```python
from build123d import *

# Parameters (mm, degrees)
F1_DEPTH      = 203.2
F1_DEPTH_BACK = 203.2
F0_W          = 63.5
F0_H          = 101.6
F0_R          = 54
F2_DEPTH      = 127
F2_DEPTH_BACK = 127
F3_DEPTH      = 101.6
F3_DEPTH_BACK = 101.6
F4_DEPTH      = 152.4
F4_DEPTH_BACK = 114.3
F5_T1_DEPTH   = 825.5
F5_T6_DEPTH   = 825.5
F5_T11_DEPTH  = 444.5
F5_T16_DEPTH  = 825.5
F5_T21_DEPTH  = 825.5
F6_DEPTH      = 152.4
F6_DEPTH_BACK = 152.4
F7_R          = 165.1
F8_DEPTH      = 50.8


# Not quite as in the source:
# - a fillet or chamfer that OpenCascade refuses, or shapes differently, is made with other operations: its cross-section is extruded or revolved along the edge and cut away or added


with BuildPart() as f1:
    # F0 (on Right) → F1 (new body, two sides)
    with BuildSketch(Plane.YZ) as f1_sk:
        Polygon((-177.8, -50.8), (-114.3, -50.8), (-114.3, 292.1), (-114.3, 330.2), (-177.8, 330.2), align=None)
    extrude(amount=F1_DEPTH)
    extrude(f1_sk.sketch, amount=-F1_DEPTH_BACK)

    # F0 (on Right) → F2 (join, two sides)
    with BuildSketch(Plane.YZ) as f2_sk:
        with BuildLine():
            ThreePointArc((-51.3464921696, -87.6703926185), (-50.5260150594, 88.1457985511), (101.6, 0))
            ThreePointArc((101.6, 0), (86.2402819365, -53.7138136006), (44.8052407181, -91.1868982047))
            Line((44.8052407181, -91.1868982047), (127, -50.8))
            Line((127, -50.8), (203.2, -50.8))
            Line((203.2, -50.8), (203.2, 203.2))
            Line((203.2, 203.2), (-25.4, 203.2))
            Line((-25.4, 203.2), (-114.3, 292.1))
            Line((-114.3, 292.1), (-114.3, -50.8))
            Line((-114.3, -50.8), (-51.3464921696, -87.6703926185))
        make_face()
        with Locations((139.7, 50.8)):
            Rectangle(F0_W, F0_H, mode=Mode.SUBTRACT)
        with BuildLine():
            ThreePointArc((44.8052407181, -91.1868982047), (86.2402819365, -53.7138136006), (101.6, 0))
            ThreePointArc((101.6, 0), (-50.5260150594, 88.1457985511), (-51.3464921696, -87.6703926185))
            ThreePointArc((-51.3464921696, -87.6703926185), (-3.7132796181, -101.5321208016), (44.8052407181, -91.1868982047))
        make_face()
        Circle(F0_R, mode=Mode.SUBTRACT)
    extrude(amount=F2_DEPTH)
    extrude(f2_sk.sketch, amount=-F2_DEPTH_BACK)

    # F0 (on Right) → F3 (join, two sides)
    with BuildSketch(Plane.YZ) as f3_sk:
        Polygon((203.2, 203.2), (203.2, -50.8), (431.8, -14.3826426938), (431.8, 162.6118868589), align=None)
    extrude(amount=F3_DEPTH)
    extrude(f3_sk.sketch, amount=-F3_DEPTH_BACK)

    # F0 (on Right) → F4 (join, two sides)
    with BuildSketch(Plane.YZ) as f4_sk:
        Circle(F0_R)
    extrude(amount=F4_DEPTH)
    extrude(f4_sk.sketch, amount=-F4_DEPTH_BACK)

    # F5: fillet of radius 152.4 on 4 edges, made by hand

    # F5_s2 → F5_t1 (cut)
    with BuildSketch(Plane.XZ.offset(-266.7)):
        with BuildLine():
            ThreePointArc((203.2, 177.8), (158.5630734528, 285.5630734528), (50.8, 330.2))
            Line((50.8, 330.2), (203.2, 330.2))
            Line((203.2, 330.2), (203.2, 177.8))
        make_face()
        with BuildLine():
            ThreePointArc((-203.2, 177.8), (-158.5630734528, 285.5630734528), (-50.8, 330.2))
            Line((-50.8, 330.2), (-203.2, 330.2))
            Line((-203.2, 330.2), (-203.2, 177.8))
        make_face()
    extrude(amount=F5_T1_DEPTH, mode=Mode.SUBTRACT)


with BuildPart() as f5_tool4:
    # F5_s5 → F5_t6 (new body)
    with BuildSketch(Plane.XZ.offset(558.8)):
        with BuildLine():
            ThreePointArc((50.8, -50.8), (158.5630734528, -6.1630734528), (203.2, 101.6))
            Line((203.2, 101.6), (203.2, -50.8))
            Line((203.2, -50.8), (50.8, -50.8))
        make_face()
    extrude(amount=-F5_T6_DEPTH)

    split(bisect_by=Plane(origin=(0, -51.3464921696, -87.6703926185), x_dir=(1, 0, 0), z_dir=(0, -0.5053788599, -0.8628975651)), keep=Keep.TOP)


with BuildPart() as f1_1:
    add(f1.part)

    # F5_t3: cut F5_tool4
    add(f5_tool4.part, mode=Mode.SUBTRACT)


with BuildPart() as f5_tool9:
    # F5_s10 → F5_t11 (new body)
    with BuildSketch(Plane.XZ.offset(558.8)):
        with BuildLine():
            ThreePointArc((50.8, -50.8), (158.5630734528, -6.1630734528), (203.2, 101.6))
            Line((203.2, 101.6), (203.2, -50.8))
            Line((203.2, -50.8), (50.8, -50.8))
        make_face()
    extrude(amount=-F5_T11_DEPTH)

    split(bisect_by=Plane.YZ.offset(127), keep=Keep.TOP)


with BuildPart() as f1_2:
    add(f1_1.part)

    # F5_t8: cut F5_tool9
    add(f5_tool9.part, mode=Mode.SUBTRACT)


with BuildPart() as f5_tool14:
    # F5_s15 → F5_t16 (new body)
    with BuildSketch(Plane.XZ.offset(558.8)):
        with BuildLine():
            ThreePointArc((-50.8, -50.8), (-158.5630734528, -6.1630734528), (-203.2, 101.6))
            Line((-203.2, 101.6), (-203.2, -50.8))
            Line((-203.2, -50.8), (-50.8, -50.8))
        make_face()
    extrude(amount=-F5_T16_DEPTH)

    split(bisect_by=Plane(origin=(0, -51.3464921696, -87.6703926185), x_dir=(1, 0, 0), z_dir=(0, -0.5053788599, -0.8628975651)), keep=Keep.TOP)


with BuildPart() as f1_3:
    add(f1_2.part)

    # F5_t13: cut F5_tool14
    add(f5_tool14.part, mode=Mode.SUBTRACT)


with BuildPart() as f5_tool19:
    # F5_s20 → F5_t21 (new body)
    with BuildSketch(Plane.XZ.offset(558.8)):
        with BuildLine():
            ThreePointArc((-50.8, -50.8), (-158.5630734528, -6.1630734528), (-203.2, 101.6))
            Line((-203.2, 101.6), (-203.2, -50.8))
            Line((-203.2, -50.8), (-50.8, -50.8))
        make_face()
    extrude(amount=-F5_T21_DEPTH)

    split(bisect_by=Plane.YZ.offset(-127), keep=Keep.BOTTOM)


with BuildPart() as f1_4:
    add(f1_3.part)

    # F5_t18: cut F5_tool19
    add(f5_tool19.part, mode=Mode.SUBTRACT)

    # F0 (on Right) → F6 (join, two sides)
    with BuildSketch(Plane.YZ) as f6_sk:
        with Locations((139.7, 50.8)):
            Rectangle(F0_W, F0_H)
    extrude(amount=F6_DEPTH)
    extrude(f6_sk.sketch, amount=-F6_DEPTH_BACK)

    # F7 (on face) → F8 (cut)
    with BuildSketch(Plane.XZ.offset(177.8)):
        with Locations((25.4, 127)):
            Circle(F7_R)
    extrude(amount=-F8_DEPTH, mode=Mode.SUBTRACT)


solid = f1_4.part
```
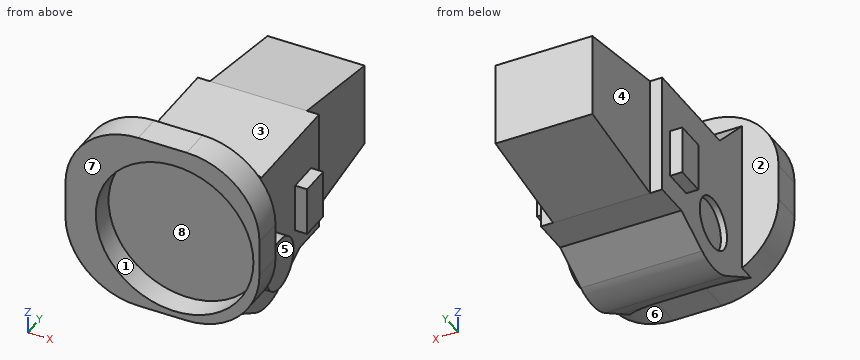
The listing builds one solid part. Answer for the finished solid, in the listing's coordinates (mm). Face numbers are marked on the shaded views. A direction names the side the tool comes from. Coordinates: 2 decimals unless noted, no trailing zeros. Loops run counter-clockwise (first coordinate to the right, second up) from the corner with the lowest first, then second, coordinate; pieces in that order, holes last. Notation, with made-up numbers: M 64,-17 L 123,-17 A18 ccw 123,6 Z; hole C 63.25,5 d5. An arc over 180 degrees is marked long. Answer as a JSON object with one key per item and string values. Group by question number.
Item 1: Section A-A (y = 0) is taken. Write down the section's boundary in (x, z).
Item 2: Which of the six approach directions +Z, -Z, +X, -X, +Y, -Y give full straight-line access (tool end or side, diameter ignored) to the marked faces 1, 2, 3, 4 and 5?
Item 3: Determine the mould class of the marked faces 6, 7 and 8 for opening direction X: +X half, -X half, draft (parallel to the pull), parting line (faces both ways), or undercut.
Item 4: Section C-C (x = 25.4) is taken. Write down the section's boundary in (y, z), and give its area (3 significant figures).
Item 5: Section B-B (z = 127) is taken. Write down the section's boundary in (x, y), and give its area (3 significant figures).
Item 6: Each of these flat-tipped pins is pushed along its axis until it touches: P1, Ø12.5, axis at x = -142, z = 40.5, coming from the +Y side; P2, Ø10, axis at x = -18.5, y = 132.5, coming from the -Z side; P3, Ø12, axis at y = 107, z = 114, coming from the -X side; P4, Ø1, axis at x = -134, y = 106, coming from the +Z side. Where does it stop, or does it pass through?
Item 7: Consider L1, parallel to Z at x = 25.4, y = -146.5; L2, parallel to Z at x = -123, y = 0; L3, parallel to X at y = 76, z = 162. Determine where each line is inside the solid, lowest interval first.
Item 8: Section D-D (y = 134) is taken. Write down the section's boundary in (x, z), and give its area (3 significant figures).
Solved:
{
 "1": {"outline": "M -127,-101.6 L 127,-101.6 L 127,-54 L 152.4,-54 L 152.4,54 L 127,54 L 127,203.2 L -127,203.2 L -127,54 L -114.3,54 L -114.3,-54 L -127,-54 Z"},
 "2": {"face 1": "-Y", "face 2": "+Z", "face 3": "+Z, +X, -X, +Y", "face 4": "+Z, -Z, -X, +Y", "face 5": "+Z, -Z, +X, +Y"},
 "3": {"face 6": "+X half", "face 7": "draft", "face 8": "undercut"},
 "4": {"outline": "M -177.8,-50.8 L -114.3,-50.8 L -51.35,-87.67 A101.6 ccw 44.81,-91.19 L 127,-50.8 L 203.2,-50.8 L 431.8,-14.38 L 431.8,162.61 L 203.2,203.2 L -25.4,203.2 L -114.3,292.1 L -114.3,330.2 L -177.8,330.2 L -177.8,292.1 L -127,292.1 L -127,-38.1 L -177.8,-38.1 Z", "area": "149,000 mm2"},
 "5": {"outline": "M -203.2,-177.8 L -139.7,-177.8 L -139.7,-127 L 190.5,-127 L 190.5,-177.8 L 203.2,-177.8 L 203.2,-114.3 L 127,-114.3 L 127,203.2 L 101.6,203.2 L 101.6,431.8 L -101.6,431.8 L -101.6,203.2 L -127,203.2 L -127,-114.3 L -203.2,-114.3 Z", "area": "136,000 mm2"},
 "6": {"P1": "stops at y = 171.45", "P2": "stops at z = -50.8", "P3": "stops at x = -127", "P4": "passes through"},
 "7": {"L1": "z = -50.8 to -38.1, 292.1 to 330.2", "L2": "z = -101.6 to -54, 54 to 203.2", "L3": "x = -127 to 127"},
 "8": {"outline": "M -152.4,0 L -127,0 L -127,-50.8 L 127,-50.8 L 127,0 L 152.4,0 L 152.4,101.6 L 127,101.6 L 127,203.2 L -127,203.2 L -127,101.6 L -152.4,101.6 Z", "area": "69,700 mm2"}
}
